from build123d import *

# Parameters (mm, degrees)
F1_DEPTH      = 300
F1_DEPTH_BACK = 300


with BuildPart() as f1:
    # F0 (on Front) → F1 (new body, two sides)
    with BuildSketch(Plane.XZ) as f1_sk:
        with BuildLine():
            Line((14.5, 7.649844), (4.472136, 4))
            ThreePointArc((4.472136, 4), (-6, 0), (4.472136, -4))
            Line((4.472136, -4), (14.5, -7.649844))
            Line((14.5, -7.649844), (14.5, -15))
            Line((14.5, -15), (17, -15))
            Line((17, -15), (17, 15))
            Line((17, 15), (14.5, 15))
            Line((14.5, 15), (14.5, 7.649844))
        make_face()
    extrude(amount=F1_DEPTH)
    extrude(f1_sk.sketch, amount=-F1_DEPTH_BACK)


solid = f1.part
Design review of the part built by this model. Coordinates are the model's own, in mm. A direction names the side the tool comes from. Give positions to 0.01 mm unless a question says otherwise; leave off trailing zeros. Loops run counter-clockwise (first coordinate to the right, second up) from the corner with the lowest first, then second, coordinate; pieces in that order, holes last. Notation, with made-up numbers: (-31.75, 24.5) -> (-5.75, 24.5) arc R26 cw to (-5.75, 57.5) -> close; hole circle Ø4 at (-11.5, 59.5). An arc over 180 degrees is marked (long way). One line per question, with ' | ' between items. Start each with the question number.
(1) We need section B-B (x = 0). State the section outline as (y, z) points, and give its area (3 significant figures).
(2) For faces 1 (the face through (9.42, -4.2, -5.8)), 2 (the face through (9.56, -4.2, 5.85)), 3 (the face through (8, 300, 0)), list the 3-axis set-ups (+Z, -Z, +X, -X, +Y, -Y) from which the entire face can be reached by the end or side of a thin tool; tool diameter is ignored.
(3) For line 1 (X direction, y = 163, z = -12); line 2 (Z direction, x = -1, y = 171.5); line 3 (X direction, y = -40.5, z = 2.5), list the stretches that pass through material, from the lowest coordinate up.
(4) Draft analysis for pull direction X (two halves, no side actions). For faces 4 (the face through (-6, -4, 0)), 5 (the face through (8, -300, 0)), 6 (the face through (17, -4, 0)), state which applies: +X half, -X half, draft (parallel to the pull), parting line (faces both ways), or undercut.
(5) We need section A-A (y = -147.5). State the section outline as (x, z) points, and give its area (3 significant figures).
(6) Insertion check: P1, Ø2, axis at y = 122, z = 10, coming from the -X side; P2, Ø4, axis at x = 11.5, y = 152.5, coming from the -Z side; P3, Ø1.5, axis at y = 193.5, z = -4.5, coming from the -X side. Each pin has a flat end and moves straight along its axis. Give the tip position at first contact, or say it passes through.
The answers:
1) outline: (-300, -6) -> (300, -6) -> (300, 6) -> (-300, 6) -> close | area: 7,200 mm^2
2) face 1: -Z, +Y, -Y | face 2: +Z, +Y, -Y | face 3: +Z, -Z, +X, -X, +Y
3) line 1: x = 14.5 to 17 | line 2: z = -5.92 to 5.92 | line 3: x = -5.45 to 17
4) face 4: undercut | face 5: draft | face 6: +X half
5) outline: (4.47, -4) -> (14.5, -7.65) -> (14.5, -15) -> (17, -15) -> (17, 15) -> (14.5, 15) -> (14.5, 7.65) -> (4.47, 4) arc R6 ccw (long way) to start | area: 297 mm^2
6) P1: stops at x = 14.5 | P2: stops at z = -7.29 | P3: stops at x = -4.68
